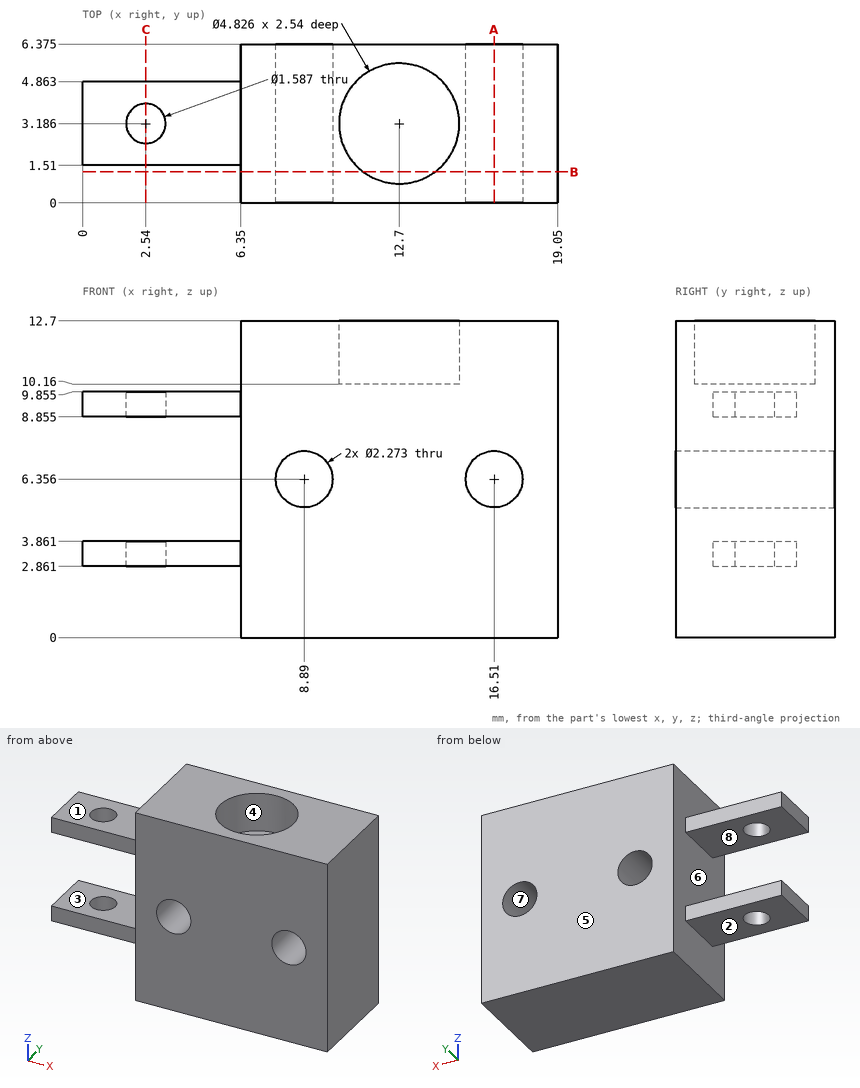
For this review, use the dimensioned drawing (mm, ordinates from the lowest corner) and the shaded views. A direction names the side the tool comes from. Give positions to 0.01 mm unless a question says otherwise; leave off trailing zeros. Write each loop counter-clockwise with the first axis right and the second up, starting at its lowest first coordinate (ties: lowest second). Pieces come first, ordered by that corner, then holes.
(1) Tool access review of the marked faces 1, 2, 3, 4 and 5: name each direction out of +Z, -Z, +X, -X, +Y, -Y from which nothing blocks a thin tool from reaching the whole face with its end or side.
(2) Consider section B-B, the plane y = 1.25. Give the boundary of the cut face in (x, z), and give its area (3 significant figures).
(3) The part is to be moulded in two halves that separate along X. For the marked faces 6, 7 and 8, say which applies: released by +X, released by -X, zero draft, split by the parting line, or undercut.
(4) To check wall thickness, follow L1, parallel to Z at x = 3.75, y = 3.25 (1 decimal); L2, parallel to X at y = 6.25, z = 6.25; L3, parallel to Y at x = 2.54, z = 3.35. State the ranges of each line that lie inside material, in increasing order.
(5) Consider section C-C, the plane x = 2.54. Give the boundary of the cut face in (y, z) (1 decimal).
(6) Consider section A-A, the plane x = 16.51. Give the boundary of the cut face in (y, z) (1 decimal).
(7) For P1, Ø2.5, axis at x = 4.5, y = 4, coming from the -Z side; P2, Ø1.1, axis at x = 2.5, z = 9, coming from the -Y side; P3, Ø1.1, axis at x = 3, z = 3, coming from the +Y side, all flat-tipped, find the tip position at first contact; note any pin that passes through.
Returned:
1. face 1: +Z, -X, +Y, -Y
1. face 2: -Z, -X, +Y, -Y
1. face 3: -X, +Y, -Y
1. face 4: +Z
1. face 5: +Z, -Z, +X, -X, +Y
2. outline: (6.35, 0) - (19.05, 0) - (19.05, 12.7) - (14.14, 12.7) - (14.14, 10.16) - (11.26, 10.16) - (11.26, 12.7) - (6.35, 12.7) - close; hole circle Ø2.27 at (8.89, 6.36); hole circle Ø2.27 at (16.51, 6.36)
2. area: 146 mm2
3. face 6: released by -X
3. face 7: undercut
3. face 8: zero draft
4. L1: z = 2.9 to 3.9, 8.9 to 9.9
4. L2: x = 6.35 to 7.76, 10.02 to 15.38, 17.64 to 19.05
4. L3: y = 1.51 to 2.39, 3.98 to 4.86
5. outline: (1.5, 2.9) - (2.4, 2.9) - (2.4, 3.9) - (1.5, 3.9) - close; (1.5, 8.9) - (2.4, 8.9) - (2.4, 9.9) - (1.5, 9.9) - close; (4, 2.9) - (4.9, 2.9) - (4.9, 3.9) - (4, 3.9) - close; (4, 8.9) - (4.9, 8.9) - (4.9, 9.9) - (4, 9.9) - close
6. outline: (0, 0) - (6.4, 0) - (6.4, 5.2) - (0, 5.2) - close; (0, 7.5) - (6.4, 7.5) - (6.4, 12.7) - (0, 12.7) - close
7. P1: stops at z = 2.86
7. P2: stops at y = 1.51
7. P3: stops at y = 4.86
